CAD build for the part. Positions are in the model's coordinates, mm. A direction names the side the tool comes from. Give positions to 0.01 mm unless a question says otherwise; leave off trailing zeros. Order: outer loops, then holes, each group sorted by start corner. A loop starts at its lowest first (then second) coordinate and runs counter-clockwise, first axis right, second up.
Item 1: Which spindle directions (+Z, -Z, +X, -X, +Y, -Y) get a long thin tool onto all of the face, cutting with end or side? Do faces 5 (the flat face through (17.8, -7.4, -7.9)), 6 (the flat face through (-9, -0.1, -3)), 7 (the flat face through (-18, -8, 9)), 8 (the flat face through (16.5, -7.5, -9)). Say none if no direction does.
Item 2: Band-saw the part on B-B on x = 14. Give the cut face in (y, z) (3 decimals).
Item 3: Band-saw the part on A-A on y = -11.5. Count the separate pieces of the cut face and the enclosed holes in it, plus the area to 3 significant figures.
Item 4: Flat gauge pins, fed straight in: P1, Ø0.6, axis at x = 4, z = -3, coming from the +Y side; P2, Ø2, axis at y = -10.5, z = 5.5, coming from the -X side; P3, Ø5, axis at x = 1.5, y = -11, coming from the -Z side; P4, Ø1.2, axis at x = -18, z = 8.5, coming from the -Y side. Where does each tip first touch, or does it go through?
Item 5: Wall check: L1, parallel to Y at x = -7, z = -7; L2, parallel to Y at x = 2, z = 6.75. Give the ranges that are in metal, low to high.
Item 6: Two-plate mould, pull along Z, no slides. Class faces 1 (the flat face through (-18.8, -4, 0)), 2 (the flat face through (0, -4, -9.5)), 3 (the flat face through (14, -0.1, -6)), 4 (the flat face through (0, -4, 9.5)): released by +Z, released by -Z, zero draft, split by the parting line, or undercut.
Item 7: Band-saw the part on C-C on z = 3.5. Give the cut face in (x, y), plus the area to 3 significant figures.
```python
from build123d import *

# Parameters (mm, degrees)
SKETCH1_W           = 37.6
SKETCH1_H           = 19
BOSS_EXTRUDE1_DEPTH = 8
SKETCH2_R           = 0.8
CUT_EXTRUDE2_DEPTH  = 0.1
LPATTERN1_COUNT     = 2
LPATTERN1_PITCH     = 12.7
LPATTERN1_COL_COUNT = 2
LPATTERN1_COL_PITCH = 12.7
SKETCH3_W           = 35.6
SKETCH3_H           = 17
CUT_EXTRUDE3_DEPTH  = 1
CUT_EXTRUDE4_REACH  = 29.901
CUT_EXTRUDE5_REACH  = 41.598
SKETCH6_R           = 0.25
BOSS_EXTRUDE2_DEPTH = 6.3


with BuildPart() as part:
    # Sketch1 → Boss-Extrude1 (new body)
    with BuildSketch(Plane(origin=(0, 0, 0), x_dir=(1, 0, 0), z_dir=(0, 1, 0))):
        Rectangle(SKETCH1_W, SKETCH1_H)
    extrude(amount=-BOSS_EXTRUDE1_DEPTH)

    # Sketch2 → Cut-Extrude2 (cut)
    with BuildSketch(Plane(origin=(0, 0, 0), x_dir=(1, 0, 0), z_dir=(0, 1, 0))):
        with Locations(Location((4.65, -6.38, 0), (0, 0, 270))):
            Circle(SKETCH2_R)
        Polygon((-1.952160074, 7.1), (3.947839926, 7.1), (4.330286309, 6.610490952), (3.300285866, 5.65), (-1.739648247, 5.65), (-2.484598632, 6.603493012), align=None)
        Polygon((-3.974480793, -7.1), (1.896221961, -7.1), (2.47230822, -6.591070163), (1.710455735, -5.65), (-3.295309805, -5.65), (-4.377887189, -6.591070163), align=None)
        Polygon((-2.436227615, 0.725), (2.588908996, 0.725), (3.190979416, 0.03239721), (2.378770347, -0.725), (-2.634272031, -0.725), (-3.228830819, 0.036000546), align=None)
        Polygon((-3.257787721, 5.920086849), (-3.95590304, 0.952738247), (-3.420237283, 0.267117343), (-2.587224094, 0.991244661), (-1.961121981, 5.446192679), (-2.706072366, 6.399685691), align=None)
        Polygon((4.918287738, 5.894984695), (4.223764825, 0.953197385), (3.436295545, 0.241486663), (2.860442223, 0.952803342), (3.485903792, 5.403193652), (4.532747216, 6.349325404), align=None)
        Polygon((-4.227399341, -0.979058314), (-4.914771822, -5.869967647), (-4.533510098, -6.3579604), (-3.492963653, -5.453427176), (-2.858633029, -0.939930263), (-3.394044886, -0.254634337), align=None)
        Polygon((3.9576888, -0.940031907), (3.272664385, -5.814233886), (2.718039978, -6.3579604), (1.96390108, -5.426418363), (2.588908996, -0.979255956), (3.398498757, -0.224301291), align=None)
    cut_extrude2 = extrude(amount=-CUT_EXTRUDE2_DEPTH, mode=Mode.SUBTRACT)

    # LPattern1: Cut-Extrude2 ×2
    with Locations(*[(-i * LPATTERN1_PITCH, 0, 0) for i in range(1, LPATTERN1_COUNT)]):
        add(cut_extrude2, mode=Mode.SUBTRACT)

    # LPattern1 col: Cut-Extrude2 ×2
    with Locations(*[(i * LPATTERN1_COL_PITCH, 0, 0) for i in range(1, LPATTERN1_COL_COUNT)]):
        add(cut_extrude2, mode=Mode.SUBTRACT)

    # Sketch3 → Cut-Extrude3 (cut)
    with BuildSketch(Plane.XZ.offset(8)):
        Rectangle(SKETCH3_W, SKETCH3_H)
    extrude(amount=-CUT_EXTRUDE3_DEPTH, mode=Mode.SUBTRACT)

    # Cut-Extrude4: up to this face of the body (flat: up to its plane)
    cut_extrude4_end = Plane(part.part.faces().sort_by_distance((0, -4, 9.5))[0])
    # Sketch4 → Cut-Extrude4 (cut, up to the picked face)
    with BuildSketch(Plane(origin=(0, 0, -9.5), x_dir=(-1, 0, 0), z_dir=(0, 0, -1)), mode=Mode.PRIVATE) as cut_extrude4_sk1:
        Polygon((-17, -8), (17, -8), (16, -7), (-16, -7), align=None)
    cut_extrude4_tool1 = split(extrude(cut_extrude4_sk1.sketch, amount=-CUT_EXTRUDE4_REACH, mode=Mode.PRIVATE), bisect_by=cut_extrude4_end, keep=Keep.BOTH, mode=Mode.PRIVATE)
    add(cut_extrude4_tool1.solids().sort_by(Axis((0, -7.505051, -9.5), (0, 0, 1)))[0], mode=Mode.SUBTRACT)

    # Cut-Extrude5: up to this face of the body (flat: up to its plane)
    cut_extrude5_end = Plane(part.part.faces().sort_by_distance((-18.8, -4, 0))[0])
    # Sketch5 → Cut-Extrude5 (cut, up to the picked face)
    with BuildSketch(Plane(origin=(18.8, 0, 0), x_dir=(0, 0, -1), z_dir=(1, 0, 0)), mode=Mode.PRIVATE) as cut_extrude5_sk1:
        Polygon((-8, -8), (8, -8), (7, -7), (-7, -7), align=None)
    cut_extrude5_tool1 = split(extrude(cut_extrude5_sk1.sketch, amount=-CUT_EXTRUDE5_REACH, mode=Mode.PRIVATE), bisect_by=cut_extrude5_end, keep=Keep.BOTH, mode=Mode.PRIVATE)
    add(cut_extrude5_tool1.solids().sort_by(Axis((18.8, -7.511111, 0), (-1, 0, 0)))[0], mode=Mode.SUBTRACT)

    # Sketch6 → Boss-Extrude2 (add)
    with BuildSketch(Plane.XZ.offset(7)):
        with Locations(Location((-6.35, -7.62, 0), (0, 0, 270))):
            Circle(SKETCH6_R)
        with Locations(Location((-3.81, -7.62, 0), (0, 0, 270))):
            Circle(SKETCH6_R)
        with Locations(Location((-1.27, -7.62, 0), (0, 0, 270))):
            Circle(SKETCH6_R)
        with Locations(Location((1.27, -7.62, 0), (0, 0, 270))):
            Circle(SKETCH6_R)
        with Locations(Location((3.81, -7.62, 0), (0, 0, 270))):
            Circle(SKETCH6_R)
        with Locations(Location((6.35, -7.62, 0), (0, 0, 270))):
            Circle(SKETCH6_R)
        with Locations(Location((-3.81, 7.62, 0), (0, 0, 270))):
            Circle(SKETCH6_R)
        with Locations(Location((-1.27, 7.62, 0), (0, 0, 270))):
            Circle(SKETCH6_R)
        with Locations(Location((1.27, 7.62, 0), (0, 0, 270))):
            Circle(SKETCH6_R)
        with Locations(Location((3.81, 7.62, 0), (0, 0, 270))):
            Circle(SKETCH6_R)
        with Locations(Location((6.35, 7.62, 0), (0, 0, 270))):
            Circle(SKETCH6_R)
        with Locations(Location((-6.35, 7.62, 0), (0, 0, 270))):
            Circle(SKETCH6_R)
    extrude(amount=BOSS_EXTRUDE2_DEPTH)


solid = part.part
```
The answers:
1. face 5: -Y
1. face 6: +Y
1. face 7: +Z, -Z, +X, -X, -Y
1. face 8: +Z, -Z, -Y
2. outline: (-7, -9.5) - (0, -9.5) - (0, -7.1) - (-0.1, -7.1) - (-0.1, -5.65) - (0, -5.65) - (0, -0.725) - (-0.1, -0.725) - (-0.1, 0.725) - (0, 0.725) - (0, 5.65) - (-0.1, 5.65) - (-0.1, 7.1) - (0, 7.1) - (0, 9.5) - (-7, 9.5) - close
3. separate pieces: 12
3. enclosed holes: 0
3. area: 2.36 mm2
4. P1: stops at y = -0.1
4. P2: passes through
4. P3: stops at z = -7.87
4. P4: stops at y = -8
5. L1: y = -7 to 0
5. L2: y = -7 to -0.1
6. face 1: zero draft
6. face 2: released by -Z
6. face 3: undercut
6. face 4: released by +Z
7. outline: (-18.8, -7) - (18.8, -7) - (18.8, 0) - (16.3, 0) - (16.3, -0.1) - (14.93, -0.1) - (14.93, 0) - (9.48, 0) - (9.48, -0.1) - (8.12, -0.1) - (8.12, 0) - (3.6, 0) - (3.6, -0.1) - (2.23, -0.1) - (2.23, 0) - (-3.22, 0) - (-3.22, -0.1) - (-4.58, -0.1) - (-4.58, 0) - (-9.1, 0) - (-9.1, -0.1) - (-10.47, -0.1) - (-10.47, 0) - (-15.92, 0) - (-15.92, -0.1) - (-17.28, -0.1) - (-17.28, 0) - (-18.8, 0) - close
7. area: 262 mm2
